Can you work these out from the model? Positions are in its coordinate system, mm. A direction names the side the tool comes from. Give positions to 0.01 mm unless a question says otherwise; leave off trailing zeros. Order: outer loops, then holes, each group sorted by start corner. A loop starts at its lowest first (then second) coordinate and runs counter-clockwise, first axis right, second up. Notation, with made-up numbers: (-8.75, 52) -> (0.25, 52) arc R29 ccw to (0.25, 80) -> close; hole circle Ø5 at (34, 34). An arc over 180 degrees is marked (long way). Answer as a JSON object with one key per item and string values.
```python
from build123d import *

# Parameters (mm, degrees)
ESQUISSE1_R             = 12.5
BOSS_EXTRU_1_DEPTH      = 80
BOSS_EXTRU_2_DEPTH      = 90
BOSS_EXTRU_2_DEPTH_BACK = 10
ESQUISSE2_R             = 2.5
CONG_1_R                = 2
CONG_2_R                = 2
ENL_V_START             = -5
ESQUISSE3_R             = 0.5
ENL_V_MAT_EXTRU_1_DEPTH = 90
ENL_V_MAT_EXTRU_2_DEPTH = 1
ENL_V_MAT_EXTRU_3_DEPTH = 1


with BuildPart() as part:
    # Esquisse1 → Boss.-Extru.1 (new body)
    with BuildSketch(Plane.XY):
        Circle(ESQUISSE1_R)
    extrude(amount=BOSS_EXTRU_1_DEPTH)

    # Esquisse2 → Boss.-Extru.2 (add, two sides: drawn at the far end of the back side and taken through both)
    with BuildSketch(Plane.XY.offset(-BOSS_EXTRU_2_DEPTH_BACK)):
        with Locations(Location((0, 0, 0), (0, 0, 180))):
            Circle(ESQUISSE2_R)
    extrude(amount=BOSS_EXTRU_2_DEPTH + BOSS_EXTRU_2_DEPTH_BACK)

    # Congé1
    cong_1_edges = [part.edges().sort_by_distance(p)[0] for p in [
        (2.5, 0, 80),
    ]]
    fillet(cong_1_edges, radius=CONG_1_R)

    # Congé2
    cong_2_edges = [part.edges().sort_by_distance(p)[0] for p in [
        (2.5, 0, 0),
    ]]
    fillet(cong_2_edges, radius=CONG_2_R)

    # Esquisse3 → Enlèv. mat.-Extru.1 (cut)
    with BuildSketch(Plane.XY.offset(90).offset(ENL_V_START)):
        Circle(ESQUISSE3_R)
    extrude(amount=-ENL_V_MAT_EXTRU_1_DEPTH, mode=Mode.SUBTRACT)

    # Esquisse4 → Enlèv. mat.-Extru.2 (cut)
    with BuildSketch(Plane(origin=(0, 0, -10), x_dir=(-1, 0, 0), z_dir=(0, 0, -1))):
        with BuildLine():
            Line((-2.449489743, -0.5), (2.449489743, -0.5))
            ThreePointArc((2.449489743, -0.5), (2.5, 0), (2.449489743, 0.5))
            Line((2.449489743, 0.5), (-2.449489743, 0.5))
            ThreePointArc((-2.449489743, 0.5), (-2.5, 0), (-2.449489743, -0.5))
        make_face()
    extrude(amount=-ENL_V_MAT_EXTRU_2_DEPTH, mode=Mode.SUBTRACT)

    # Esquisse5 → Enlèv. mat.-Extru.3 (cut)
    with BuildSketch(Plane.XY.offset(90)):
        with BuildLine():
            Line((-2.449489743, -0.5), (2.449489743, -0.5))
            ThreePointArc((2.449489743, -0.5), (2.5, 0), (2.449489743, 0.5))
            Line((2.449489743, 0.5), (-2.449489743, 0.5))
            ThreePointArc((-2.449489743, 0.5), (-2.5, 0), (-2.449489743, -0.5))
        make_face()
    extrude(amount=-ENL_V_MAT_EXTRU_3_DEPTH, mode=Mode.SUBTRACT)


solid = part.part
```
1. If we section it at C-C on x = -10.5: Please give me the cut outline in (y, z), then the cut area to 3 significant figures.
Worked answers:
{"outline": "(-6.78, 0) -> (6.78, 0) -> (6.78, 80) -> (-6.78, 80) -> close", "area": "1,090 mm²"}
2. If we section it at A-A on z = 53.5: Please give me the cut outline in (x, y), then the cut area to 3 significant figures.
Worked answers:
{"outline": "circle Ø25 at (0, 0); hole circle Ø1 at (0, 0)", "area": "490 mm²"}
3. For faces 1 (the face through (0, -5, 80)), 2 (the face through (-2.385, -0.751, -6.056)), 3 (the face through (0, -1, 90)), which set-ups out of +Z, -Z, +X, -X, +Y, -Y let a thin tool reach every point of the face, with its end or its side?
Worked answers:
{"face 1": "+Z", "face 2": "-Z", "face 3": "+Z, +X, -X, +Y, -Y"}
4. Will these pins go through, and if not, where does the flat tip stop? pin 1 Ø3 at (x, y) = (0.5, 5) entering from +Z; pin 2 Ø4 at (x, z) = (9.5, 73.5) entering from -Y; pin 3 Ø1 at (x, z) = (-7.5, 38) entering from +Y.
Worked answers:
{"pin 1": "z = 80.25", "pin 2": "y = -10", "pin 3": "y = 10.36"}
5. If we section it at B-B on x = 10: Please give me the cut outline in (y, z).
Worked answers:
{"outline": "(-7.5, 0) -> (7.5, 0) -> (7.5, 80) -> (-7.5, 80) -> close"}
6. Please list where these lines run through material, in increasing order: L1, parallel to Y at x = 0, z = 40; L2, parallel to Z at x = 4, y = 8.25; L3, parallel to X at y = 10, z = 8.
Worked answers:
{"L1": "-12.5 to -0.5, 0.5 to 12.5", "L2": "0 to 80", "L3": "-7.5 to 7.5"}
